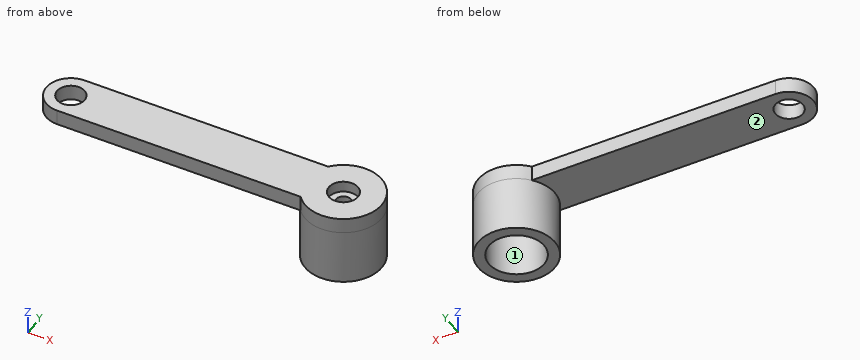
from build123d import *

# Parameters (mm, degrees)
SKETCH_1_R          = 4.5
EXTRUDE_1_DEPTH     = 5
EXTRUDE_START       = 18
SKETCH_4_R          = 12.5
EXTRUDE_3_DEPTH     = 18
SKETCH_5_R          = 9
CUT_EXTRUDE_1_DEPTH = 15
CUT_EXTRUDE_2_REACH = 72.2
SKETCH_6_R          = 2.5
SKETCH_7_R          = 4.75
CUT_EXTRUDE_3_DEPTH = 3.6


with BuildPart() as part:
    # 草图1 → 凸台-拉伸1 (new body)
    with BuildSketch(Plane.XY):
        with BuildLine():
            Line((-37.363516522, 8), (43.031797122, 8))
            ThreePointArc((43.031797122, 8), (65.136483478, 0), (43.031797122, -8))
            Line((43.031797122, -8), (-37.363516522, -8))
            ThreePointArc((-37.363516522, -8), (-45.363516522, 0), (-37.363516522, 8))
        make_face()
        with Locations((-37.363516522, 0)):
            Circle(SKETCH_1_R, mode=Mode.SUBTRACT)
    extrude(amount=EXTRUDE_1_DEPTH)

    # 草图4 → 凸台-拉伸3 (add)
    with BuildSketch(Plane(origin=(0, 0, 0), x_dir=(-1, 0, 0), z_dir=(0, 0, -1)).offset(EXTRUDE_START)):
        with Locations((-52.636483478, 0)):
            Circle(SKETCH_4_R)
    extrude(amount=-EXTRUDE_3_DEPTH)

    # 草图5 → 切除-拉伸1 (cut)
    with BuildSketch(Plane(origin=(0, 0, -18), x_dir=(-1, 0, 0), z_dir=(0, 0, -1))):
        with Locations((-52.636483478, 0)):
            Circle(SKETCH_5_R)
    extrude(amount=-CUT_EXTRUDE_1_DEPTH, mode=Mode.SUBTRACT)

    # 草图6 → 切除-拉伸2 (cut, up to next)
    with BuildSketch(Plane.XY.offset(5), mode=Mode.PRIVATE) as cut_extrude_2_sk1:
        with Locations((52.636483478, 0)):
            Circle(SKETCH_6_R)
    cut_extrude_2_tool1 = extrude(cut_extrude_2_sk1.sketch, amount=-CUT_EXTRUDE_2_REACH, mode=Mode.PRIVATE) & part.part
    add(cut_extrude_2_tool1.solids().sort_by_distance((52.636483, 0, 5))[0], mode=Mode.SUBTRACT)

    # 草图7 → 切除-拉伸3 (cut)
    with BuildSketch(Plane.XY.offset(5)):
        with Locations((52.636483478, 0)):
            Circle(SKETCH_7_R)
    extrude(amount=-CUT_EXTRUDE_3_DEPTH, mode=Mode.SUBTRACT)


solid = part.part
Design review of the part built by this model. Coordinates are the model's own, in mm. Face numbers are marked on the shaded views. Round coordinates to 2 decimals unless told otherwise and drop trailing zeros. Write each loop counter-clockwise with the first axis right and the second up, starting at its lowest first coordinate (ties: lowest second). Pieces come first, ordered by that corner, then holes. Notation, with made-up numbers: M -12,78.5 L 25,78.5 A18 cw 25,95.5 Z; hole C 2.25,26 d8. An arc over 180 degrees is marked long. One line per item, written item: value. Start each with the question number.
1. Take a section at A-A on y = 0. State the section outline as (x, z) points, then the cut area to 3 significant figures.
2. Take a section at B-B on x = 53. State the section outline as (y, z) points, then the cut area to 3 significant figures.
3. Clearance check with flat-ended pins moving along their axes: P1, Ø8, axis at x = 15, y = -2, coming from the -Z side; P2, Ø10, axis at x = 36.5, z = -3.5, coming from the +Y side; P3, Ø12.5, axis at x = 52.64, y = 0, coming from the -Z side. State where each tip first meets the part, or that it passes through.
4. Take a section at D-D on y = -6. State the section outline as (x, z) points, then the cut area to 3 significant figures.
5. Draft analysis for pull direction X (two halves, no side actions). For the marked faces 1 and 2, state which applies: pulls with the +X half, pulls with the -X half, needs draft (parallel to the pull), parting line crosses it, or undercut.
6. To check wall thickness, follow probe 1 along X at (y, z) = (-3.25, 2); probe 2 along Y at (x, z) = (11, 2.5); probe 3 along Z at (x, y) = (55, 4.5). State the ranges of each line that lie inside material, in increasing order. Write a range as from..to.
7. Take a section at C-C on z = -7.75. State the section outline as (x, y) points, then the cut area to 3 significant figures.
Computed:
1. outline: M -45.36,0 L -41.86,0 L -41.86,5 L -45.36,5 Z; M -32.86,0 L 40.14,0 L 40.14,-18 L 43.64,-18 L 43.64,-3 L 50.14,-3 L 50.14,1.4 L 47.89,1.4 L 47.89,5 L -32.86,5 Z; M 55.14,-3 L 61.64,-3 L 61.64,-18 L 65.14,-18 L 65.14,5 L 57.39,5 L 57.39,1.4 L 55.14,1.4 Z
1. area: 631 mm²
2. outline: M -12.49,-18 L -8.99,-18 L -8.99,-3 L -2.47,-3 L -2.47,1.4 L -4.74,1.4 L -4.74,5 L -12.49,5 Z; M 2.47,-3 L 8.99,-3 L 8.99,-18 L 12.49,-18 L 12.49,5 L 4.74,5 L 4.74,1.4 L 2.47,1.4 Z
2. area: 249 mm²
3. P1: stops at z = 0
3. P2: stops at y = 8
3. P3: stops at z = -3
4. outline: M -42.66,0 L 41.67,0 L 41.67,-18 L 45.93,-18 L 45.93,-3 L 59.34,-3 L 59.34,-18 L 63.6,-18 L 63.6,5 L -42.66,5 Z
4. area: 725 mm²
5. face 1: undercut
5. face 2: needs draft
6. probe 1: x = -44.67..-40.48, -34.25..49.17, 56.1..64.71
6. probe 2: y = -8..8
6. probe 3: z = -3..5
7. outline: C 52.64,0 d25; hole C 52.64,0 d18
7. area: 236 mm²
